from build123d import *

# Parameters (mm, degrees)
F0_W      = 30
F0_H      = 22.8446739912
F1_DEPTH  = 30
F3_DEPTH  = 50.001
F5_DEPTH  = 50.001
F6_W      = 20.5
F6_H      = 18
F7_DEPTH  = 30.001
F8_W      = 23.6850994825
F8_H      = 6.8956923813
F9_DEPTH  = 50.001
F11_DEPTH = 50.001
F12_W     = 22.8446739912
F12_H     = 2.6407527924
F13_DEPTH = 40.0010001


with BuildPart() as f1:
    # F0 (on Top) → F1 (new body)
    with BuildSketch(Plane.XY):
        with BuildLine():
            ThreePointArc((25, 0), (0, 25), (-25, 0))
            Line((-25, 0), (-25, -45))
            Line((-25, -45), (-15, -45))
            Line((-15, -45), (15, -45))
            Line((15, -45), (25, -45))
            Line((25, -45), (25, 0))
        make_face()
        with Locations((0, -56.4223369956)):
            Rectangle(F0_W, F0_H)
    extrude(amount=F1_DEPTH)

    # F2 (on face) → F3 (cut, through all)
    with BuildSketch(Plane(origin=(-25, 0, 0), x_dir=(0, -1, 0), z_dir=(-1, 0, 0))):
        Polygon((0, 0), (0, 6.8956923813), (-25.6583113223, 19.2217491567), (-25.6583113223, 0), align=None)
        Polygon((0, 0), (14.3542923033, 0), (0, 6.8956923813), align=None)
    extrude(amount=-F3_DEPTH, mode=Mode.SUBTRACT)

    # F4 (on face) → F5 (cut, through all)
    with BuildSketch(Plane(origin=(-25, 0, 0), x_dir=(0, -1, 0), z_dir=(-1, 0, 0))):
        Polygon((-22.0570550542, 27.4019237886), (-22.0570550542, 30), (-24.7225984931, 30), align=None)
        Polygon((-19.0570550542, 24.8038475773), (-16.0570550542, 30), (-22.0570550542, 30), align=None)
        Polygon((-13.0570550542, 24.8038475773), (-10.0570550542, 30), (-16.0570550542, 30), align=None)
        Polygon((-7.0570550542, 24.8038475773), (-4.0570550542, 30), (-10.0570550542, 30), align=None)
        Polygon((-1.0570550542, 24.8038475773), (0, 26.6347206375), (0, 30), (-4.0570550542, 30), align=None)
        Polygon((0, 30), (0, 26.6347206375), (1.9429449458, 30), align=None)
        Polygon((4.9429449458, 24.8038475773), (7.9429449458, 30), (1.9429449458, 30), align=None)
        Polygon((10.9429449458, 24.8038475773), (13.9429449458, 30), (7.9429449458, 30), align=None)
        Polygon((16.9429449458, 24.8038475773), (19.9429449458, 30), (13.9429449458, 30), align=None)
        Polygon((22.9429449458, 24.8038475773), (25.9429449458, 30), (19.9429449458, 30), align=None)
        Polygon((28.9429449458, 24.8038475773), (31.9429449458, 30), (25.9429449458, 30), align=None)
        Polygon((34.9429449458, 24.8038475773), (37.9429449458, 30), (31.9429449458, 30), align=None)
        Polygon((40.9429449458, 24.8038475773), (43.9429449458, 30), (37.9429449458, 30), align=None)
    extrude(amount=-F5_DEPTH, mode=Mode.SUBTRACT)

    # F6 (on Top) → F7 (cut, through all)
    with BuildSketch(Plane.XY):
        with BuildLine():
            ThreePointArc((14.0728856666, 16.9101711705), (8.1838650627, 20.4211741248), (1.5, 21.9488040676))
            Line((1.5, 21.9488040676), (1.5, 16.9101711705))
            Line((1.5, 16.9101711705), (14.0728856666, 16.9101711705))
        make_face()
        with BuildLine():
            ThreePointArc((-1.5, 21.9488040676), (-8.1838650627, 20.4211741248), (-14.0728856666, 16.9101711705))
            Line((-14.0728856666, 16.9101711705), (-1.5, 16.9101711705))
            Line((-1.5, 16.9101711705), (-1.5, 21.9488040676))
        make_face()
        with BuildLine():
            Line((1.5, 14.8383843921), (1.5, 0))
            Line((1.5, 0), (22, 0))
            ThreePointArc((22, 0), (20.5102096408, 7.9580965369), (16.2426090463, 14.8383843921))
            Line((16.2426090463, 14.8383843921), (1.5, 14.8383843921))
        make_face()
        with BuildLine():
            ThreePointArc((-16.2426090463, 14.8383843921), (-20.5102096408, 7.9580965369), (-22, 0))
            Line((-22, 0), (-1.5, 0))
            Line((-1.5, 0), (-1.5, 14.8383843921))
            Line((-1.5, 14.8383843921), (-16.2426090463, 14.8383843921))
        make_face()
        with Locations((-11.75, -12)):
            Rectangle(F6_W, F6_H)
        with Locations((-11.75, -33)):
            Rectangle(F6_W, F6_H)
        with Locations((11.75, -12)):
            Rectangle(F6_W, F6_H)
        with Locations((11.75, -33)):
            Rectangle(F6_W, F6_H)
    extrude(amount=F7_DEPTH, mode=Mode.SUBTRACT)

    # F8 (on face) → F9 (cut, through all)
    with BuildSketch(Plane(origin=(-25, 0, 0), x_dir=(0, -1, 0), z_dir=(-1, 0, 0))):
        with Locations((56.8425497413, 3.4478461906)):
            Rectangle(F8_W, F8_H)
        Polygon((0, 6.8956923813), (14.3542923033, 0), (45, 0), (45, 6.8956923813), align=None)
    extrude(amount=-F9_DEPTH, mode=Mode.SUBTRACT)

    # F10 (on face) → F11 (cut, through all)
    with BuildSketch(Plane(origin=(-25, 0, 0), x_dir=(0, -1, 0), z_dir=(-1, 0, 0))):
        with BuildLine():
            add(Edge.make_bspline(
                [(-25.4602208734, 21.6052159667), (-1.3237191597, 14.7319072857), (24.7841980308, 12.3858377337), (45, 12.1211158112)],
                knots=[0, 0, 0, 0, 71.0956460079, 71.0956460079, 71.0956460079, 71.0956460079], degree=3))
            Line((-25.4602208734, 21.6052159667), (-25.4602208734, 18.728017807))
            Line((-25.4602208734, 18.728017807), (0, 6.8956923813))
            Line((0, 6.8956923813), (45, 6.8956923813))
            Line((45, 6.8956923813), (45, 12.1211158112))
        make_face()
    extrude(amount=-F11_DEPTH, mode=Mode.SUBTRACT)

    # F12 (on face) → F13 (cut, through all)
    with BuildSketch(Plane(origin=(-15, 0, 0), x_dir=(0, -1, 0), z_dir=(-1, 0, 0))):
        with Locations((56.4223369956, 28.6796236038)):
            Rectangle(F12_W, F12_H)
        Polygon((67.8446739912, 15.5053976923), (45, 15.5053976923), (45, 12.1211158112), (45, 6.8956923813), (67.8446739912, 6.8956923813), align=None)
    extrude(amount=-F13_DEPTH, mode=Mode.SUBTRACT)


solid = f1.part
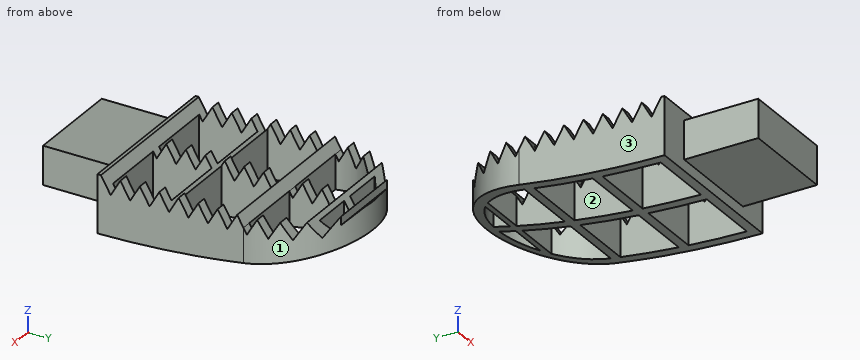
For this review, take the finished solid that the model builds, in its own axes (mm). Face numbers are marked on the shaded views. Round coordinates to 2 decimals unless told otherwise and drop trailing zeros. Order: outer loops, then holes, each group sorted by start corner. A loop starts at its lowest first (then second) coordinate and runs counter-clockwise, first axis right, second up. Notation, with made-up numbers: M 32,1.25 L 57,1.25 A14 cw 57,6.25 Z; hole C -38.75,35.25 d4. An arc over 180 degrees is marked long. Write each question's results on one line, items separated by ' | '. Start each with the question number.
1. To check wall thickness, follow L1, parallel to Y at x = -8, z = 17; L2, parallel to X at y = -32, z = 18.25; L3, parallel to Y at x = 19, z = 20.5. State the ranges of each line that lie inside material, in increasing order. Write a range as [from, to].
2. Clearance check with flat-ended pins moving along their axes: pin 1 Ø3 at (y, z) = (-58, 18) entering from +X; pin 2 Ø7 at (y, z) = (10.5, 24) entering from +X; pin 3 Ø1.5 at (x, z) = (15.5, 14) entering from -Y. State where each tip first meets the part, or that it passes through.
3. Add section A-A (y = -48). State the section outline as (x, z) points, then the cut area to 3 significant figures.
4. Draft analysis for pull direction Y (two halves, no side actions). For the marked faces 1, 2 and 3, state which applies: pulls with the +Y half, pulls with the -Y half, needs draft (parallel to the pull), parting line crosses it, or undercut.
5. Add section B-B (x = -9). State how many separate pieces and enclosed holes the cut face has, then the cut area to 3 significant figures.
Output values:
1) L1: [-67.84, -42], [-24, -21], [-3, 0] | L2: [-25, -22], [-1.5, 1.5], [22, 25] | L3: [-45, -42], [-24, -21], [-3, 0], [11.09, 16.25]
2) pin 1: x = 15 | pin 2: x = 24 | pin 3: y = -45
3) outline: M -15,15.51 L 15,15.51 L 15,27.36 L -15,27.36 Z | area: 356 mm^2
4) face 1: pulls with the +Y half | face 2: undercut | face 3: needs draft
5) separate pieces: 5 | enclosed holes: 0 | area: 444 mm^2
